Part model, mm, in its own coordinate system. A direction names the side the tool comes from. Give positions to 0.01 mm unless a question says otherwise; leave off trailing zeros. Write each loop counter-clockwise with the first axis right and the second up, starting at its lowest first coordinate (ties: lowest second). Pieces come first, ordered by that corner, then holes. Notation, with made-up numbers: M 76,54 L 121,54 A22 cw 121,66 Z; hole C -34.75,-29 d4. An arc over 180 degrees is marked long. Use a Markdown table: item, result. Add a question column.
from build123d import *

# Parameters (mm, degrees)
SKETCH1_R           = 6.35
BOSS_EXTRUDE1_DEPTH = 38.1


with BuildPart() as part:
    # Sketch1 → Boss-Extrude1 (new body)
    with BuildSketch(Plane(origin=(0, 0, 0), x_dir=(0, 0, -1), z_dir=(1, 0, 0))):
        with Locations(Location((0, 0, 0), (0, 0, 180))):
            Circle(SKETCH1_R)
    extrude(amount=BOSS_EXTRUDE1_DEPTH)

    # Sketch4 → Tap Drill for 1/4-20 Tap1 (revolve, cut)
    with BuildSketch(Plane.ZX):
        Polygon((0, 0), (0, 14.233816902), (2.5527, 12.7), (2.5527, 0), align=None)
    tap_drill_for_1_4_20_tap1 = revolve(axis=Axis((-6.35, 0, 0), (1, 0, 0)), mode=Mode.SUBTRACT)

    # Mirror1: Tap Drill for 1/4-20 Tap1 across plane
    add(tap_drill_for_1_4_20_tap1.mirror(Plane.ZY.offset(-19.05)), mode=Mode.SUBTRACT)


solid = part.part
1. Flat gauge pins, fed straight in: pin 1 (6 mm diameter, centred on y = 0, z = 0, fed in from -X); pin 2 (5 mm diameter, centred on x = 29.5, z = 4, fed in from -Y). Where does each tip first touch, or does it go through?
2. Tool access for faces 1 (the conical face through (13.97, 0.43, -0.1)), 2 (the cylindrical face through (31.839, -0.767, 2.435)): list every direction of +Z, -Z, +X, -X, +Y, -Y with a clear straight run to the whole face (end or side of a thin tool).
3. Cut at C-C (z = -3.25). Write the cut outline in (x, y).
4. Cut at D-D (z = 4). Write the cut outline in (x, y).
5. Mould opens along Y. For faces 3 (the conical face through (24.13, 0.43, -0.1)), 4 (the cylindrical face through (18.783, 5.634, 2.93)), 5 (the cylindrical face through (6.261, -0.767, 2.435)), 6 (the flat face through (38.1, 0, 3)) say: released by +Y, released by -Y, zero draft, split by the parting line, or undercut.
6. Cut at B-B (x = 23). Write the cut outline in (y, z).
7. Drill centre lines: probe 1 along Y at (x, z) = (28, 0); probe 2 along Z at (x, y) = (10, -1.25); probe 3 along Y at (x, z) = (30.5, 1.75). Where is each one in solid material? Low to high. Write a range as [from, to].
8. Cut at A-A (x = 10). Write the cut outline in (y, z), then the cut area to 3 significant figures.
A:
| question | item | result |
|---|---|---|
| 1 | pin 1 | stops at x = 0 |
| 1 | pin 2 | stops at y = -6.17 |
| 2 | face 1 | -X |
| 2 | face 2 | +X |
| 3 | outline | M 0,-5.46 L 38.1,-5.46 L 38.1,5.46 L 0,5.46 Z |
| 4 | outline | M 0,-4.93 L 38.1,-4.93 L 38.1,4.93 L 0,4.93 Z |
| 5 | face 3 | undercut |
| 5 | face 4 | split by the parting line |
| 5 | face 5 | undercut |
| 5 | face 6 | zero draft |
| 6 | outline | C 0,0 d12.7 |
| 7 | probe 1 | y = [-6.35, -2.55], [2.55, 6.35] |
| 7 | probe 2 | z = [-6.23, -2.23], [2.23, 6.23] |
| 7 | probe 3 | y = [-6.1, -1.86], [1.86, 6.1] |
| 8 | outline | C 0,0 d12.7; hole C 0,0 d5.11 |
| 8 | area | 106 mm² |
